For this review, take the finished solid that the model builds, in its own axes (mm). Face numbers are marked on the shaded views. A direction names the side the tool comes from. Give positions to 0.01 mm unless a question says otherwise; leave off trailing zeros. Order: outer loops, then holes, each group sorted by start corner. A loop starts at its lowest first (then second) coordinate and runs counter-clockwise, first axis right, second up. Notation, with made-up numbers: (61.25, 45) -> (93.25, 45) arc R17 cw to (93.25, 63) -> close; hole circle Ø2 at (26, 31.25). An arc over 180 degrees is marked (long way). Return JSON: item names as keys, results as strings. Group by question number.
1) For the marked faces 1 and 2, list the 3-axis set-ups (+Z, -Z, +X, -X, +Y, -Y) from which the entire face can be reached by the end or side of a thin tool; tool diameter is ignored.
2) Insertion check: P1, Ø23.5, axis at x = 21.5, z = 36, coming from the -Y side; P2, Ø1.6, axis at y = 41, z = 28, coming from the -X side; P3, Ø10.5, axis at y = 21, z = 25, coming from the +X side; P4, Ø6, axis at x = 6, y = 21.5, coming from the -Z side. Each pin has a flat end and moves straight along its axis. Give the tip position at first contact, or say it passes through.
3) Add section C-C (z = 33). Give the boundary of the cut face in (x, y).
4) Add section D-D (y = 33.5). Give the boundary of the cut face in (x, z).
5) Add section A-A (z = 25). Give the boundary of the cut face in (x, y).
6) Add section B-B (y = 21). Give the boundary of the cut face in (x, z), then the cut area to 3 significant figures.
7) To check wall thickness, follow line 1 along X through (y, z) = (10, 18); line 2 along Y through (x, z) = (28.5, 24); line 3 along Y through (x, z) = (0.8, 25). State the ranges of each line that lie inside material, in increasing order.
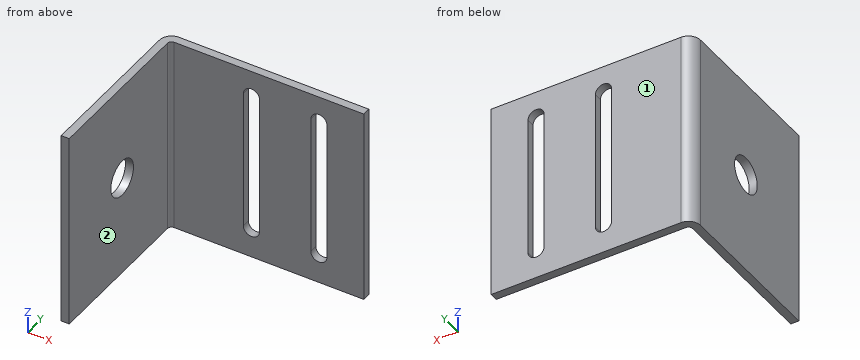
from build123d import *

# Parameters (mm, degrees)
BASE_FLANGE1_DEPTH = 49
SKETCH7_R          = 4.5
CUT_EXTRUDE1_DEPTH = 82.639451248
CUT_EXTRUDE2_DEPTH = 82.639451248


# Sheet-metal steps are written as plain solids
with BuildPart() as part:
    # Sketch1 → Base-Flange1 (new body)
    with BuildSketch(Plane.XY):
        with BuildLine():
            Line((0, 0), (0, 39))
            ThreePointArc((0, 39), (0.878679656, 41.121320344), (3, 42))
            Line((3, 42), (50, 42))
            Line((50, 42), (50, 40))
            Line((50, 40), (3, 40))
            ThreePointArc((3, 40), (2.292893219, 39.707106781), (2, 39))
            Line((2, 39), (2, 0))
            Line((2, 0), (0, 0))
        make_face()
    extrude(amount=BASE_FLANGE1_DEPTH)

    # Sketch7 → Cut-Extrude1 (cut, through all)
    with BuildSketch(Plane.ZY):
        with Locations((25, 21)):
            Circle(SKETCH7_R)
    extrude(amount=-CUT_EXTRUDE1_DEPTH, mode=Mode.SUBTRACT)

    # Sketch6 → Cut-Extrude2 (cut, through all)
    with BuildSketch(Plane(origin=(0, 42, 0), x_dir=(1, 0, 0), z_dir=(0, 1, 0))):
        with BuildLine():
            Line((40.874848709, -7.388922921), (40.874848709, -42.388922921))
            ThreePointArc((40.874848709, -42.388922921), (38.874848709, -44.388922921), (36.874848709, -42.388922921))
            Line((36.874848709, -42.388922921), (36.874848709, -7.388922921))
            ThreePointArc((36.874848709, -7.388922921), (38.874848709, -5.388922921), (40.874848709, -7.388922921))
        make_face()
        with BuildLine():
            Line((20.163393388, -7.388922921), (20.163393388, -42.388922921))
            ThreePointArc((20.163393388, -42.388922921), (22.163393388, -44.388922921), (24.163393388, -42.388922921))
            Line((24.163393388, -42.388922921), (24.163393388, -7.388922921))
            ThreePointArc((24.163393388, -7.388922921), (22.163393388, -5.388922921), (20.163393388, -7.388922921))
        make_face()
    extrude(amount=-CUT_EXTRUDE2_DEPTH, mode=Mode.SUBTRACT)


solid = part.part
Evaluation:
{
 "1": {"face 1": "+Z, -Z, +X, -X, +Y", "face 2": "+Z, -Z, +X, -Y"},
 "2": {"P1": "y = 40", "P2": "x = 0.25", "P3": "x = 2", "P4": "through"},
 "3": {"outline": "(0, 0) -> (2, 0) -> (2, 39) arc R1 cw to (3, 40) -> (20.16, 40) -> (20.16, 42) -> (3, 42) arc R3 ccw to (0, 39) -> close; (24.16, 40) -> (36.87, 40) -> (36.87, 42) -> (24.16, 42) -> close; (40.87, 40) -> (50, 40) -> (50, 42) -> (40.87, 42) -> close"},
 "4": {"outline": "(0, 0) -> (2, 0) -> (2, 49) -> (0, 49) -> close"},
 "5": {"outline": "(0, 0) -> (2, 0) -> (2, 16.5) -> (0, 16.5) -> close; (0, 25.5) -> (2, 25.5) -> (2, 39) arc R1 cw to (3, 40) -> (20.16, 40) -> (20.16, 42) -> (3, 42) arc R3 ccw to (0, 39) -> close; (24.16, 40) -> (36.87, 40) -> (36.87, 42) -> (24.16, 42) -> close; (40.87, 40) -> (50, 40) -> (50, 42) -> (40.87, 42) -> close"},
 "6": {"outline": "(0, 0) -> (2, 0) -> (2, 20.5) -> (0, 20.5) -> close; (0, 29.5) -> (2, 29.5) -> (2, 49) -> (0, 49) -> close", "area": "80.0 mm^2"},
 "7": {"line 1": "0 to 2", "line 2": "40 to 42", "line 3": "0 to 16.5, 25.5 to 41.04"}
}
